Can you work these out from the drawing? Everything is in mm from the part's minimum corner. A direction names the side the tool comes from. Coordinates: 2 decimals unless noted, no trailing zeros. Loops run counter-clockwise (first coordinate to the right, second up) from the corner with the lowest first, then second, coordinate; pieces in that order, holes last. Notation, with made-up numbers: (-39.75, -34.5) -> (-25.75, -34.5) arc R10 ccw to (-25.75, -16.5) -> close; hole circle Ø11 at (-10, -22). An arc over 180 degrees is marked (long way). One line per question, with ' | ' between items.
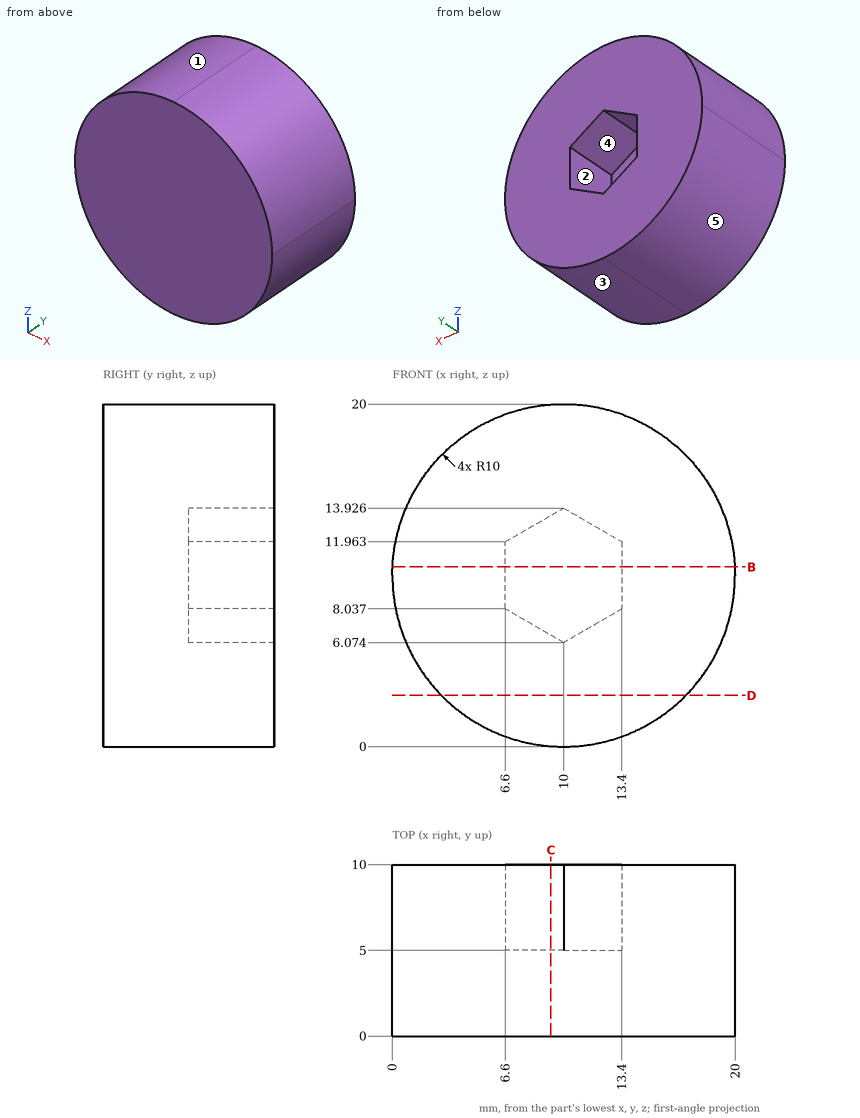
Q1. For pin 1 (1.5 mm diameter, centred on y = 2, z = 17.5, fed in from +X); pin 2 (1.5 mm diameter, centred on y = 4, z = 3, fed in from -X); pin 3 (4 mm diameter, centred on x = 16.5, z = 4, fed in from -Y); pin 4 (6 mm diameter, centred on y = 3, z = 17.5, fed in from -X), each with a flat end and sliding along its axis, tell me the tip position at first contact or that it passes through.
Values follow:
pin 1: stops at x = 17.38 | pin 2: stops at x = 2.19 | pin 3: stops at y = 0 | pin 4: stops at x = 1.07
Q2. Imagine slicing it at D-D on z = 3. Write out the boundary of the cut face in (x, y).
Values follow:
outline: (2.86, 0) -> (17.14, 0) -> (17.14, 10) -> (2.86, 10) -> close
Q3. Imagine slicing it at C-C on x = 9.25. Write out the boundary of the cut face in (y, z).
Values follow:
outline: (0, 0.03) -> (10, 0.03) -> (10, 6.51) -> (5, 6.51) -> (5, 13.49) -> (10, 13.49) -> (10, 19.97) -> (0, 19.97) -> close
Q4. Please list where these lines run through material, in increasing order: L1, parallel to Z at x = 13.25, y = 9.5; L2, parallel to X at y = 8.75, z = 8 (1 decimal); L3, parallel to X at y = 5.75, z = 13.25. Write a range as [from, to].
Values follow:
L1: z = [0.54, 7.95], [12.05, 19.46] | L2: x = [0.2, 6.7], [13.3, 19.8] | L3: x = [0.54, 8.83], [11.17, 19.46]
Q5. We'd pull the mould along X, two halves only. Please class the marked faces 3, 4 and 5: released by +X, released by -X, zero draft, split by the parting line, or undercut.
Values follow:
face 3: released by +X | face 4: undercut | face 5: released by -X
Q6. For the marked faces 1 and 2, which set-ups out of +Z, -Z, +X, -X, +Y, -Y let a thin tool reach every point of the face, with its end or its side?
Values follow:
face 1: +Z, -X, +Y, -Y | face 2: +Y
Q7. Imagine slicing it at B-B on z = 10.5. Write out the boundary of the cut face in (x, y).
Values follow:
outline: (0.01, 0) -> (19.99, 0) -> (19.99, 10) -> (13.4, 10) -> (13.4, 5) -> (6.6, 5) -> (6.6, 10) -> (0.01, 10) -> close
